Verification items for this drawing (mm, ordinates from the low corner). Round coordinates to 2 decimals unless told otherwise and drop trailing zeros. Loops run counter-clockwise (first coordinate to the right, second up) from the corner with the lowest first, then second, coordinate; pieces in that order, holes last. Notation, with made-up numbers: (-27, 8.5) - (10, 8.5) arc R21 ccw to (10, 32.5) - close; hole circle Ø2 at (4.25, 23). An arc over 180 degrees is marked (long way). Write item = value, one per line.
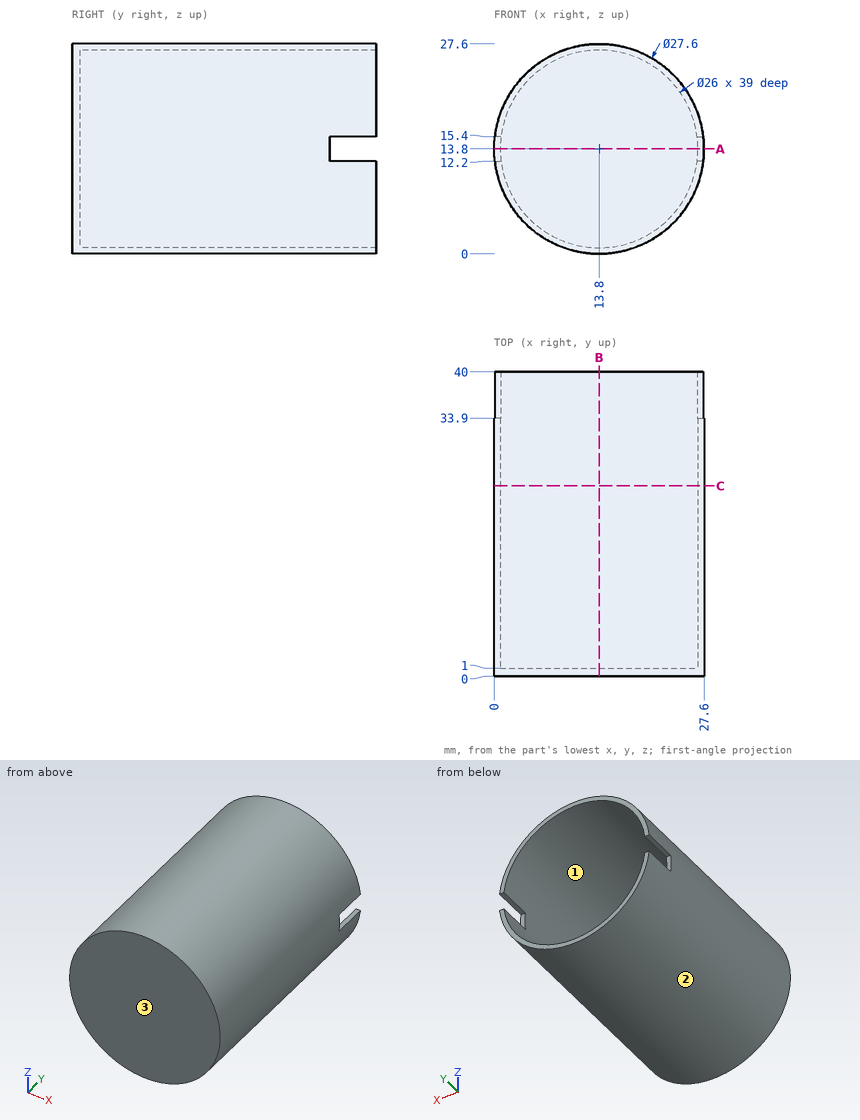
(1) Section check B-B (x = 13.8). Enter the section's corners in (y, z), then the cut area to 3 significant figures.
Answers follow:
outline = (0, 0) - (40, 0) - (40, 0.8) - (1, 0.8) - (1, 26.8) - (40, 26.8) - (40, 27.6) - (0, 27.6) - close
area = 90.0 mm²
(2) Mould release check, pull along Z, two halves, no side actions. Record for the marked faces 1, 2 and 3: pulls with the +Z half, pulls with the -Z half, needs draft (parallel to the pull), parting line crosses it, or undercut.
Answers follow:
face_1 = undercut
face_2 = parting line crosses it
face_3 = needs draft
(3) Section check C-C (y = 25). Enter the section's corners in (x, z).
Answers follow:
outline = circle Ø27.6 at (13.8, 13.8); hole circle Ø26 at (13.8, 13.8)
(4) Section check A-A (z = 13.8). Enter the section's corners in (x, y), then the cut area to 3 significant figures.
Answers follow:
outline = (0, 0) - (27.6, 0) - (27.6, 33.9) - (26.8, 33.9) - (26.8, 1) - (0.8, 1) - (0.8, 33.9) - (0, 33.9) - close
area = 80.2 mm²
(5) Gauge pin test, flat ends, axial feed: pin 1 (6 mm diameter, centred on y = 10, z = 23.5, fed in from -X); pin 2 (3 mm diameter, centred on y = 31, z = 11.5, fed in from -X); pin 3 (3 mm diameter, centred on x = 19.5, z = 16, fed in from +Y). Record the tip position at first contact, or that the pin passes through.
Answers follow:
pin_1 = 1.74
pin_2 = 0.02
pin_3 = 1
(6) Scan lines: L1, parallel to Z at x = 13.8, y = 19; L2, parallel to Z at x = 19.75, y = 29.5. Record each from-to range of solid material in increasing order. Write a range as [from, to].
Answers follow:
L1 = [0, 0.8], [26.8, 27.6]
L2 = [1.35, 2.24], [25.36, 26.25]
